Check sheet for the modelled part. Datum: model origin and axes. Units: mm. A direction names the side the tool comes from. Round coordinates to 2 decimals unless told otherwise and drop trailing zeros. Write each loop counter-clockwise with the first axis right and the second up, starting at its lowest first coordinate (ties: lowest second). Pieces come first, ordered by that corner, then holes. Notation, with made-up numbers: (18, -7) -> (33, -7) arc R10 ccw to (33, 12) -> close; hole circle Ø9 at (23.25, -18.5). An arc over 180 degrees is marked (long way). One line per item, written item: value.
from build123d import *

# Parameters (mm, degrees)
SKETCH_1_W          = 28
SKETCH_1_H          = 17.2
EXTRUDE_1_DEPTH     = 1.5
SKETCH_2_W          = 8.2
SKETCH_2_H          = 8.34
EXTRUDE_2_DEPTH     = 2.56
SKETCH_3_R          = 0.5
CUT_EXTRUDE_1_DEPTH = 10
SKETCH_4_W          = 1.5
SKETCH_4_H          = 12.2
CUT_EXTRUDE_2_DEPTH = 10


with BuildPart() as part:
    # Sketch 1 → Extrude 1 (new body)
    with BuildSketch(Plane(origin=(0, 0, 0), x_dir=(1, 0, 0), z_dir=(0, 1, 0))):
        with Locations((14, -8.6)):
            Rectangle(SKETCH_1_W, SKETCH_1_H)
    extrude(amount=EXTRUDE_1_DEPTH)

    # Sketch 2 → Extrude 2 (add)
    with BuildSketch(Plane(origin=(0, 1.5, 0), x_dir=(1, 0, 0), z_dir=(0, 1, 0))):
        with Locations((2.5, -8.6)):
            Rectangle(SKETCH_2_W, SKETCH_2_H)
    extrude(amount=EXTRUDE_2_DEPTH)

    # Sketch 3 → Cut-Extrude 1 (cut)
    with BuildSketch(Plane(origin=(0, 1.5, 0), x_dir=(1, 0, 0), z_dir=(0, 1, 0))):
        with Locations(Location((1.8, -1.6, 0), (0, 0, 270))):
            Circle(SKETCH_3_R)
        with Locations(Location((1.8, -15.6, 0), (0, 0, 270))):
            Circle(SKETCH_3_R)
        with Locations(Location((24.8, -1.6, 0), (0, 0, 270))):
            Circle(SKETCH_3_R)
        with Locations(Location((24.8, -4.14, 0), (0, 0, 270))):
            Circle(SKETCH_3_R)
        with Locations(Location((24.8, -13.06, 0), (0, 0, 270))):
            Circle(SKETCH_3_R)
        with Locations(Location((24.8, -15.6, 0), (0, 0, 270))):
            Circle(SKETCH_3_R)
    extrude(amount=-CUT_EXTRUDE_1_DEPTH, mode=Mode.SUBTRACT)

    # Sketch 4 → Cut-Extrude 2 (cut)
    with BuildSketch(Plane(origin=(0, 1.5, 0), x_dir=(1, 0, 0), z_dir=(0, 1, 0))):
        with Locations((27.25, -8.6)):
            Rectangle(SKETCH_4_W, SKETCH_4_H)
    extrude(amount=-CUT_EXTRUDE_2_DEPTH, mode=Mode.SUBTRACT)


solid = part.part
Item 1: Sectioned sample at C-C on y = 1.05. Enter the section's corners in (x, z).
Answer:
outline: (0, 0) -> (28, 0) -> (28, 2.5) -> (26.5, 2.5) -> (26.5, 14.7) -> (28, 14.7) -> (28, 17.2) -> (0, 17.2) -> close; hole circle Ø1 at (1.8, 1.6); hole circle Ø1 at (1.8, 15.6); hole circle Ø1 at (24.8, 1.6); hole circle Ø1 at (24.8, 4.14); hole circle Ø1 at (24.8, 13.06); hole circle Ø1 at (24.8, 15.6)
Item 2: Tool access check on faces 5 (the flat face through (26.5, 1, 9)), 6 (the flat face through (-1, 1.5, 9)), 7 (the flat face through (6.6, 3, 9)). Record the directions out of +Z, -Z, +X, -X, +Y, -Y that give a thin tool (end or side, any length) a straight path to the whole face; none if there is none.
Answer:
face 5: +X, +Y, -Y
face 6: +Z, -Z, -X, -Y
face 7: +Z, -Z, +X, +Y
Item 3: Sectioned sample at B-B on x = 1.8. Enter the section's corners in (y, z).
Answer:
outline: (0, 0) -> (1.5, 0) -> (1.5, 1.1) -> (0, 1.1) -> close; (0, 2.1) -> (1.5, 2.1) -> (1.5, 4.43) -> (4.06, 4.43) -> (4.06, 12.77) -> (1.5, 12.77) -> (1.5, 15.1) -> (0, 15.1) -> close; (0, 16.1) -> (1.5, 16.1) -> (1.5, 17.2) -> (0, 17.2) -> close
Item 4: Thickness scan on line 1 (X direction, y = 0.35, z = 1.6); line 2 (X direction, y = 0.5, z = 4.14); line 3 (X direction, y = 1.05, z = 15.25). Record the ranges inside material, lowest first.
Answer:
line 1: x = 0 to 1.3, 2.3 to 24.3, 25.3 to 28
line 2: x = 0 to 24.3, 25.3 to 26.5
line 3: x = 0 to 1.44, 2.16 to 24.44, 25.16 to 28
Item 5: Sectioned sample at D-D on z = 1.6. Enter the section's corners in (x, y).
Answer:
outline: (0, 0) -> (1.3, 0) -> (1.3, 1.5) -> (0, 1.5) -> close; (2.3, 0) -> (24.3, 0) -> (24.3, 1.5) -> (2.3, 1.5) -> close; (25.3, 0) -> (28, 0) -> (28, 1.5) -> (25.3, 1.5) -> close
Item 6: Mould release check, pull along X, two halves, no side actions. Record for faces 1 (the flat face through (28, 1, 16)), 2 (the cylindrical face through (25.3, 0.8, 4.1)), 3 (the flat face through (0, 1, 9)), 4 (the flat face through (2, 3, 12.77)): pulls with the +X half, pulls with the -X half, needs draft (parallel to the pull), parting line crosses it, or undercut.
Answer:
face 1: pulls with the +X half
face 2: undercut
face 3: pulls with the -X half
face 4: needs draft
Item 7: Sectioned sample at A-A on z = 4.14. Enter the section's corners in (x, y), and give its area (4 significant figures).
Answer:
outline: (0, 0) -> (24.3, 0) -> (24.3, 1.5) -> (0, 1.5) -> close; (25.3, 0) -> (26.5, 0) -> (26.5, 1.5) -> (25.3, 1.5) -> close
area: 38.25 mm^2
Item 8: Depth check by flat-ended pin: P1, Ø2, axis at y = 3.5, z = 12, coming from the +X side; P2, Ø1.2, axis at y = 0.5, z = 10.5, coming from the -X side; P3, Ø0.5, axis at x = -0.5, z = 10, coming from the -Y side. Enter the tip coordinate at first touch or a pass-through.
Answer:
P1: stops at x = 6.6
P2: stops at x = 0
P3: stops at y = 1.5
